Design review of the part built by this model. Coordinates are the model's own, in mm. A direction names the side the tool comes from. Coordinates: 2 decimals unless noted, no trailing zeros. Order: outer loops, then holes, each group sorted by start corner. A loop starts at its lowest first (then second) coordinate and runs counter-clockwise, first axis right, second up. Notation, with made-up numbers: M 79.5,-35 L 90.5,-35 A12 ccw 90.5,-24 Z; hole C 51.25,70 d4. An arc over 180 degrees is marked long. Answer as a JSON object with one key per item and string values.
from build123d import *

# Parameters (mm, degrees)
F1_DEPTH       = 22
F3_D           = 6
F5_D           = 1.5
F5_CBORE_D     = 4
F5_CBORE_DEPTH = 2


with BuildPart() as f1:
    # F0 (on Front) → F1 (new body)
    with BuildSketch(Plane.XZ):
        Polygon((-13, 0), (0, 0), (0, 2.5), (-10, 2.5), (-10, 20), (-20, 20), (-20, 16), (-13, 16), align=None)
    extrude(amount=F1_DEPTH)

    # F3 (through all)
    with Locations(Plane.XY.offset(2.5)):
        with Locations((-6, -11)):
            Hole(F3_D / 2)

    # F5 (through all)
    with Locations(Plane.XY.offset(20)):
        with Locations((-16, -11.594802)):
            CounterBoreHole(F5_D / 2, F5_CBORE_D / 2, F5_CBORE_DEPTH)


solid = f1.part
1) Add section A-A (x = -6). State the section outline as (y, z) points.
Taken from the geometry:
{"outline": "M -22,0 L -14,0 L -14,2.5 L -22,2.5 Z; M -8,0 L 0,0 L 0,2.5 L -8,2.5 Z"}
2) Add section D-D (x = -16). State the section outline as (y, z) points, and give its area (3 significant figures).
Taken from the geometry:
{"outline": "M -22,16 L -12.34,16 L -12.34,18 L -13.59,18 L -13.59,20 L -22,20 Z; M -10.84,16 L 0,16 L 0,20 L -9.59,20 L -9.59,18 L -10.84,18 Z", "area": "77.0 mm2"}
3) Insertion check: pin 1 Ø4 at (y, z) = (-12, 8.5) entering from +X; pin 2 Ø3.5 at (x, y) = (-17.5, -7.5) entering from -Z; pin 3 Ø7 at (x, y) = (-6, -11) entering from +Z; pin 4 Ø3 at (x, y) = (-13, -8) entering from -Z. Each pin has a flat end and moves straight along its axis. Give the tip position at first contact, or say it passes through.
Taken from the geometry:
{"pin 1": "stops at x = -10", "pin 2": "stops at z = 16", "pin 3": "stops at z = 2.5", "pin 4": "stops at z = 0"}
4) Mouldability with a two-part tool opening along X and no side actions: class faces 1 (the flat face through (-17, -11, 16)), 2 (the flat face through (-13, -11, 8)), 3 (the cylindrical face through (-7.61, -8.47, 1.23)) as released by +X, released by -X, zero draft, split by the parting line, or undercut.
Taken from the geometry:
{"face 1": "zero draft", "face 2": "released by -X", "face 3": "undercut"}
5) Tool access review of faces 4 (the flat face through (-12, 0, 10)), 5 (the flat face through (-2.7, -10.8, 2.5)), 6 (the cylindrical face through (-17.59, -12.81, 19.01)): name each direction out of +Z, -Z, +X, -X, +Y, -Y from which nothing blocks a thin tool from reaching the whole face with its end or side.
Taken from the geometry:
{"face 4": "+Z, -Z, +X, -X, +Y", "face 5": "+Z, +X, +Y, -Y", "face 6": "+Z"}
6) Add section C-C (y = -17.75). State the section outline as (x, z) points.
Taken from the geometry:
{"outline": "M -20,16 L -13,16 L -13,0 L 0,0 L 0,2.5 L -10,2.5 L -10,20 L -20,20 Z"}
7) Add section B-B (y = -8.75). State the section outline as (x, z) points.
Taken from the geometry:
{"outline": "M -20,16 L -13,16 L -13,0 L -7.98,0 L -7.98,2.5 L -10,2.5 L -10,20 L -20,20 Z; M -4.02,0 L 0,0 L 0,2.5 L -4.02,2.5 Z"}
8) To check wall thickness, follow L1, parallel to Y at x = -6, z = 1.1; L2, parallel to Z at x = -5, y = -14; L3, parallel to X at y = -2, z = 3.25. State the ranges of each line that lie inside material, in increasing order.
Taken from the geometry:
{"L1": "y = -22 to -14, -8 to 0", "L2": "z = 0 to 2.5", "L3": "x = -13 to -10"}
